Can you work these out from the model? Positions are in its coordinate system, mm. Face numbers are marked on the shaded views. A direction names the side the tool comes from. Round coordinates to 2 decimals unless told otherwise and drop trailing zeros. Order: outer loops, then holes, each group sorted by start corner. A loop starts at its lowest first (then second) coordinate and runs counter-clockwise, first axis right, second up. Notation, with made-up numbers: (70, 63) -> (120, 63) arc R18 cw to (120, 90) -> close; hole circle Ø7 at (-28.5, 83.25). An arc over 180 degrees is marked (long way). Use a Markdown table: item, result. Add a question column.
Q1. If we section it at A-A on z = 0: List the corners of the cut face in (x, y) for me.
Q2. I'm going to push a flat-ended pin straight in: pin 1 Ø1 at (x, y) = (-0.5, 5.5) entering from +Z. Where does the tip first touch, or does it pass through?
Q3. For the marked faces 1 and 2, which set-ups out of +Z, -Z, +X, -X, +Y, -Y let a thin tool reach every point of the face, with its end or its side?
Q4. I need wall thicknesses on line 1 along Z through (x, y) = (0.1, 17.75); line 2 along Y through (x, z) = (1.2, -0.05); line 3 along X through (y, z) = (10.5, -0.5). Which ranges of each line are inside material? Lowest first, please. Write a range as [from, to].
Q5. If we section it at B-B on y = 24.5: List the corners of the cut face in (x, z) for me.
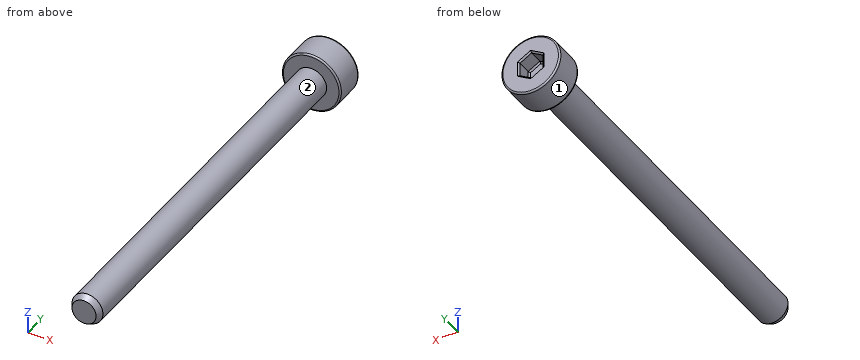
```python
from build123d import *

# Parameters (mm, degrees)
SKETCH1_R           = 1
BOSS_EXTRUDE1_DEPTH = 25
SKETCH2_R           = 1.9
BOSS_EXTRUDE2_DEPTH = 2
CUT_EXTRUDE1_DEPTH  = 1
FILLET1_R           = 0.1
CHAMFER1_SIZE       = 0.1
CHAMFER2_SIZE       = 0.1
CUT_EXTRUDE2_DEPTH  = 0.1
CUT_EXTRUDE2_DRAFT  = -45


with BuildPart() as part:
    # Sketch1 → Boss-Extrude1 (new body)
    with BuildSketch(Plane(origin=(0, 0, 0), x_dir=(1, 0, 0), z_dir=(0, 1, 0))):
        with Locations(Location((0, 0, 0), (0, 0, 270))):
            Circle(SKETCH1_R)
    extrude(amount=BOSS_EXTRUDE1_DEPTH)

    # Sketch2 → Boss-Extrude2 (add)
    with BuildSketch(Plane(origin=(0, 25, 0), x_dir=(1, 0, 0), z_dir=(0, 1, 0))):
        with Locations(Location((0, 0, 0), (0, 0, 270))):
            Circle(SKETCH2_R)
    extrude(amount=BOSS_EXTRUDE2_DEPTH)

    # Sketch3 → Cut-Extrude1 (cut)
    with BuildSketch(Plane(origin=(0, 27, 0), x_dir=(1, 0, 0), z_dir=(0, 1, 0))):
        Polygon((0, 0.866025404), (-0.75, 0.433012702), (-0.75, -0.433012702), (0, -0.866025404), (0.75, -0.433012702), (0.75, 0.433012702), align=None)
    extrude(amount=-CUT_EXTRUDE1_DEPTH, mode=Mode.SUBTRACT)

    # Fillet1
    fillet1_edges = [part.edges().sort_by_distance(p)[0] for p in [
        (0, 25, -1.9),
        (0, 27, -1.9),
    ]]
    fillet(fillet1_edges, radius=FILLET1_R)

    # Chamfer1
    chamfer1_edges = [part.edges().sort_by_distance(p)[0] for p in [
        (0, 0, -1),
    ]]
    chamfer(chamfer1_edges, length=CHAMFER1_SIZE)

    # Sketch4 → Cut-Revolve1 (revolve, cut)
    with BuildSketch(Plane.XY, mode=Mode.PRIVATE) as cut_revolve1_sk:
        Polygon((1.01, 0), (1.01, 0.4), (0.779059892, 0), align=None)
    revolve(cut_revolve1_sk.sketch.rotate(Axis((0, 0, 0), (0, 1, 0)), 180), axis=Axis((0, 0, 0), (0, 1, 0)), mode=Mode.SUBTRACT)

    # Chamfer2
    chamfer2_edges = [part.edges().sort_by_distance(p)[0] for p in [
        (0.375, 27, -0.649519053),
        (-0.375, 27, -0.649519053),
        (-0.75, 27, 0),
        (-0.375, 27, 0.649519053),
        (0.375, 27, 0.649519053),
        (0.75, 27, 0),
    ]]
    chamfer(chamfer2_edges, length=CHAMFER2_SIZE)


with BuildPart() as cut_extrude2_tool:
    # Sketch6 → Cut-Extrude2 (with draft: the straight prism first)
    with BuildSketch(Plane(origin=(0, 26, 0), x_dir=(1, 0, 0), z_dir=(0, 1, 0))):
        Polygon((0, 0.866025404), (-0.75, 0.433012702), (-0.75, -0.433012702), (0, -0.866025404), (0.75, -0.433012702), (0.75, 0.433012702), align=None)
    extrude(amount=-CUT_EXTRUDE2_DEPTH)
    # Cut-Extrude2: the draft: its side faces are tilted about the plane it starts from
    cut_extrude2_sides = [cut_extrude2_tool.faces().sort_by_distance(p)[0] for p in [
        (-0.375, 25.95, -0.649519053),
        (-0.75, 25.95, 0),
        (-0.375, 25.95, 0.649519053),
        (0.375, 25.95, 0.649519053),
        (0.75, 25.95, 0),
        (0.375, 25.95, -0.649519053),
    ]]
    draft(cut_extrude2_sides, Plane(origin=(0, 26, 0), x_dir=(1, 0, 0), z_dir=(0, 1, 0)), CUT_EXTRUDE2_DRAFT)


with BuildPart() as part_1:
    add(part.part)

    # Cut-Extrude2: cut by cut_extrude2_tool
    add(cut_extrude2_tool.part, mode=Mode.SUBTRACT)


solid = part_1.part
```
Answer below:
| question | item | result |
|---|---|---|
| 1 | outline | (-1.9, 25.1) arc R0.1 ccw to (-1.8, 25) -> (-1, 25) -> (-1, 0.38) -> (-0.78, 0) -> (0.78, 0) -> (1, 0.38) -> (1, 25) -> (1.8, 25) arc R0.1 ccw to (1.9, 25.1) -> (1.9, 26.9) arc R0.1 ccw to (1.8, 27) -> (0.85, 27) -> (0.75, 26.9) -> (0.75, 26) -> (0.65, 25.9) -> (-0.65, 25.9) -> (-0.75, 26) -> (-0.75, 26.9) -> (-0.85, 27) -> (-1.8, 27) arc R0.1 ccw to (-1.9, 26.9) -> close |
| 2 | pin 1 | z = 1 |
| 3 | face 1 | +Y, -Y |
| 3 | face 2 | -Y |
| 4 | line 1 | [-0.99, 0.99] |
| 4 | line 2 | [25, 27] |
| 4 | line 3 | [-0.87, 0.87] |
| 5 | outline | circle Ø2 at (0, 0) |
